```python
from build123d import *

# Parameters (mm, degrees)
BOSS_EXTRUDE1_DEPTH = 1.5
FILLET1_R           = 3
CHAMFER1_SIZE       = 1


with BuildPart() as part:
    # Sketch1 → Boss-Extrude1 (new body)
    with BuildSketch(Plane(origin=(0, 0, 0), x_dir=(1, 0, 0), z_dir=(0, 1, 0))):
        Polygon((0, 0), (0, 5), (10, 5), (10, 30), (-10, 30), (-10, 0), align=None)
    extrude(amount=BOSS_EXTRUDE1_DEPTH)

    # Fillet1
    fillet1_edges = [part.edges().sort_by_distance(p)[0] for p in [
        (-10, 0.75, -30),
        (10, 0.75, -30),
    ]]
    fillet(fillet1_edges, radius=FILLET1_R)

    # Chamfer1
    chamfer1_edges = [part.edges().sort_by_distance(p)[0] for p in [
        (-10, 0.75, 0),
        (10, 0.75, -5),
        (0, 0.75, 0),
    ]]
    chamfer(chamfer1_edges, length=CHAMFER1_SIZE)


solid = part.part
```
Design review of the part built by this model. Coordinates are the model's own, in mm. A direction names the side the tool comes from. Round coordinates to 2 decimals unless told otherwise and drop trailing zeros. Write each loop counter-clockwise with the first axis right and the second up, starting at its lowest first coordinate (ties: lowest second). Pieces come first, ordered by that corner, then holes.
Item 1: We need section C-C on z = -2.25. Write out the cut boundary in (x, y), and give its area (3 significant figures).
Item 2: We need section A-A on y = 0.9. Write out the cut boundary in (x, z), and give its area (3 significant figures).
Item 3: We need section B-B on x = 1.5. Write out the cut boundary in (y, z).
Item 4: For probe 1 along Z at (x, y) = (0.75, 1.1); probe 2 along X at (y, z) = (0.3, -3.5); probe 3 along Z at (x, y) = (-0.25, 0.95), list the stretches that pass through material, from the lowest coordinate up.
Item 5: For faces 1 (the flat face through (0, 1, -3)), 2 (the flat face through (-10, 1, -14)), list the 3-axis set-ups (+Z, -Z, +X, -X, +Y, -Y) from which the entire face can be reached by the end or side of a thin tool; tool diameter is ignored.
Returned:
1. outline: (-10, 0) - (0, 0) - (0, 1.5) - (-10, 1.5) - close
1. area: 15.0 mm2
2. outline: (-10, -27) arc R3 ccw to (-7, -30) - (7, -30) arc R3 ccw to (10, -27) - (10, -6) - (9, -5) - (0, -5) - (0, -1) - (-1, 0) - (-9, 0) - (-10, -1) - close
2. area: 545 mm2
3. outline: (0, -30) - (1.5, -30) - (1.5, -5) - (0, -5) - close
4. probe 1: z = -30 to -5
4. probe 2: x = -10 to 0
4. probe 3: z = -30 to -0.75
5. face 1: +Z, +X, +Y, -Y
5. face 2: +Z, -Z, -X, +Y, -Y
